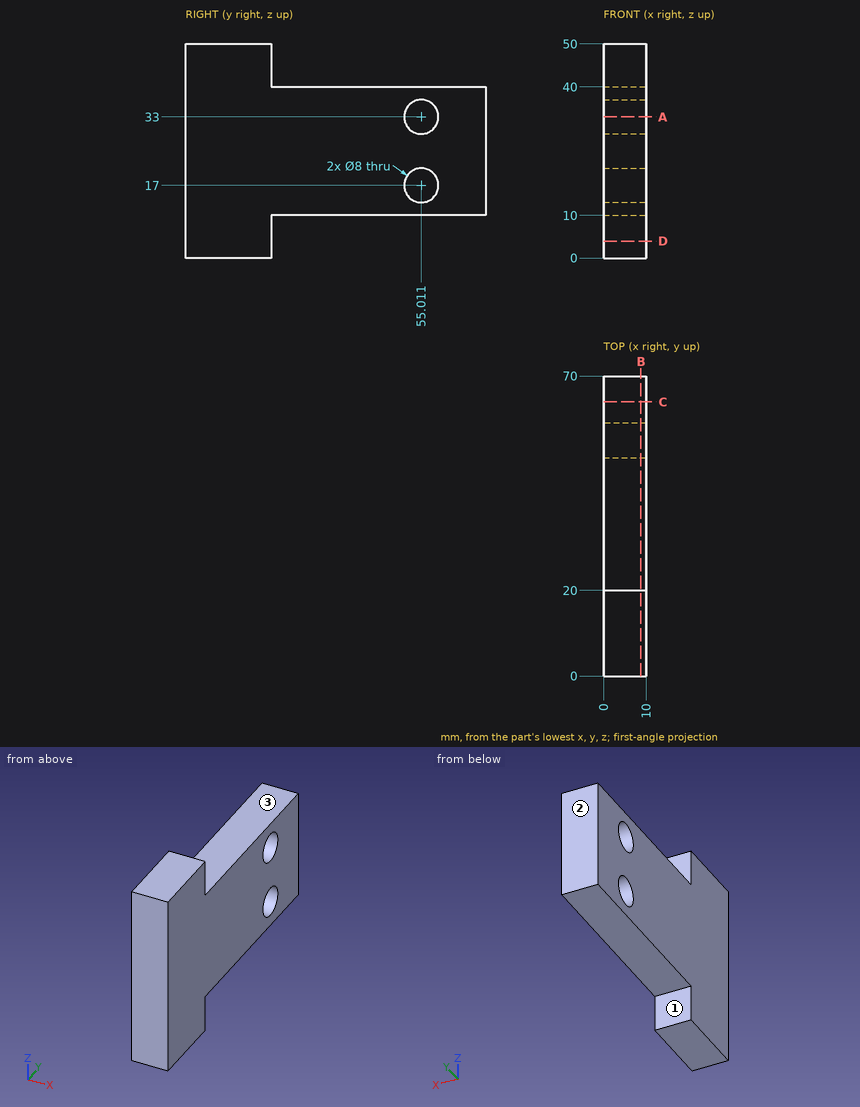
Here's the drawing with two shaded views (mm, measured from the low corner). I have some questions. A direction names the side the tool comes from. Give positions to 0.01 mm unless a question says otherwise; leave off trailing zeros. Order: outer loops, then holes, each group sorted by start corner. A loop starts at its lowest first (then second) coordinate and runs counter-clockwise, first axis right, second up. Notation, with made-up numbers: M 7.25,-20.75 L 40.25,-20.75 A29 cw 40.25,10.25 Z; hole C 58.25,16 d6. An arc over 180 degrees is marked long. Answer as a JSON object with one key per item and string values. Group by question number.
1) On a 3-axis mill with a long thin cutter (end or side, diameter ignored), from which of +Z, -Z, +X, -X, +Y, -Y can I reach the whole of each face in a straight line? I mean the marked faces 1, 2 and 3. Say none if no direction works.
2) Suppose I cut it at D-D, the plane z = 4. Write out the boundary of the cut face in (x, y).
3) Suppose I cut it at C-C, the plane y = 64. Write out the boundary of the cut face in (x, z).
4) I'm going to push flat-ended pins straight in: pin 1 Ø3 at (x, y) = (3, 44.5) entering from -Z; pin 2 Ø5 at (x, z) = (6, 44.5) entering from +Y; pin 3 Ø3 at (x, y) = (6, 34) entering from +Z. Where does each tip first touch, or does it pass through?
5) Suppose I cut it at A-A, the plane z = 33. Write out the boundary of the cut face in (x, y), plus the area to 3 significant figures.
6) Please list where these lines run through material, in increasing order: L1, parallel to Z at x = 5.5, y = 34; L2, parallel to Y at x = 8.25, z = 42. Write a range as [from, to].
7) Suppose I cut it at B-B, the plane x = 8.75. Write out the boundary of the cut face in (y, z), plus the area to 3 significant figures.
Results found:
{
 "1": {"face 1": "-Z, +X, -X, +Y", "face 2": "+Z, -Z, +X, -X, +Y", "face 3": "+Z, +X, -X, +Y"},
 "2": {"outline": "M 0,0 L 10,0 L 10,20 L 0,20 Z"},
 "3": {"outline": "M 0,10 L 10,10 L 10,40 L 0,40 Z"},
 "4": {"pin 1": "z = 10", "pin 2": "y = 20", "pin 3": "z = 40"},
 "5": {"outline": "M 0,0 L 10,0 L 10,51.01 L 0,51.01 Z; M 0,59.01 L 10,59.01 L 10,70 L 0,70 Z", "area": "620 mm²"},
 "6": {"L1": "[10, 40]", "L2": "[0, 20]"},
 "7": {"outline": "M 0,0 L 20,0 L 20,10 L 70,10 L 70,40 L 20,40 L 20,50 L 0,50 Z; hole C 55.01,17 d8; hole C 55.01,33 d8", "area": "2,400 mm²"}
}
